The drawing under review shows one solid part. Ordinate dimensions are in mm from its lowest x, y, z. A direction names the side the tool comes from. Round coordinates to 2 decimals unless told otherwise and drop trailing zeros. Write each loop counter-clockwise with the first axis right and the second up, starting at its lowest first coordinate (ties: lowest second). Pieces come first, ordered by that corner, then holes.
Item 1: Machinability: for the marked faces 1 and 2, which of the approach directions +Z, -Z, +X, -X, +Y, -Y give a long, thin tool a straight path to every point of the face, cutting with its end or side? Answer none if there is none.
Item 2: Draft analysis for pull direction X (two halves, no side actions). For the marked faces 3, 4 and 5, state which applies: +X half, -X half, draft (parallel to the pull), parting line (faces both ways), or undercut.
Item 3: Clearance check with a flat-ended pin moving along its axis: pin 1 Ø0.8 at (y, z) = (12, 1.5) entering from +X. State where the tip first meets the part, or that it passes through.
Item 4: To check wall thickness, follow L1, parallel to Y at x = 4.5, z = 1.45; L2, parallel to Y at x = 4, z = 2; L3, parallel to X at y = 16.5, z = 1.35. State the ranges of each line that lie inside material, in increasing order.
Item 5: Add section A-A (x = 2.5). Give the boundary of the cut face in (y, z).
Item 6: Add section C-C (y = 14.5). Give the boundary of the cut face in (x, z).
Item 7: Add section B-B (z = 1.35). Give the boundary of the cut face in (x, y) (3 decimals).
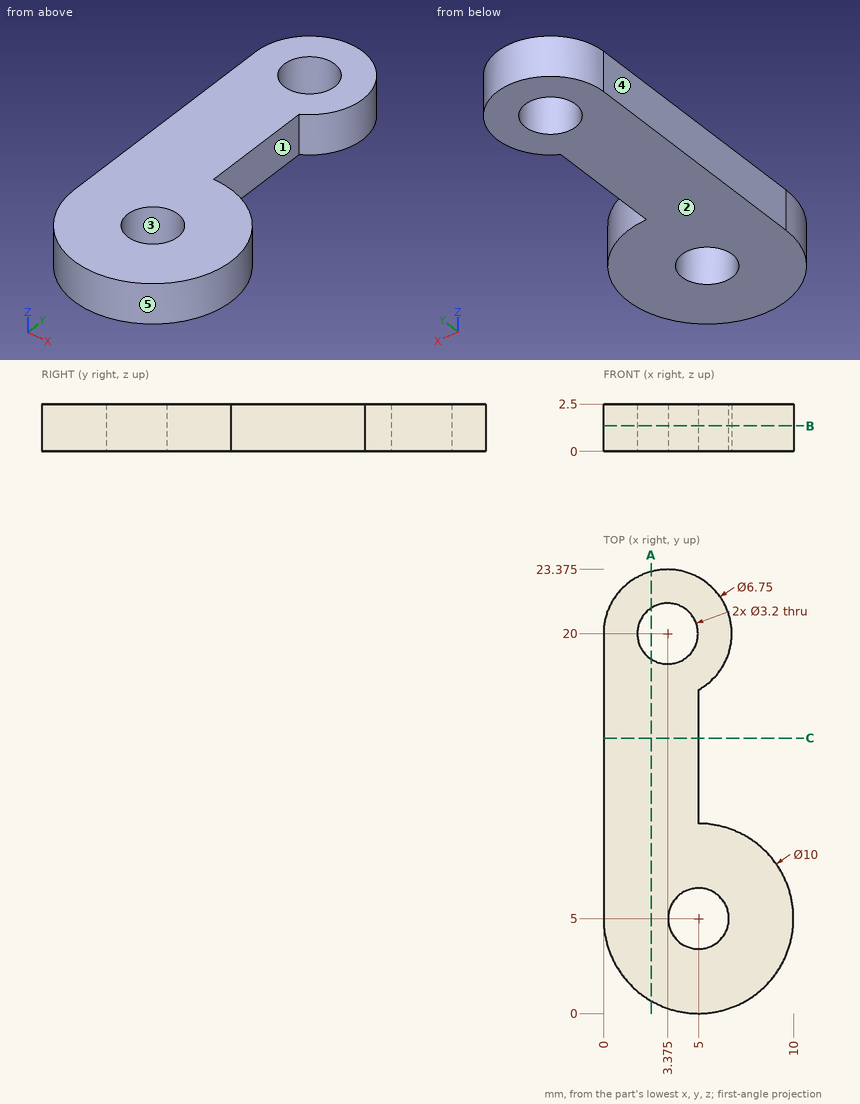
Numbers:
1. face 1: +Z, -Z, +X
1. face 2: -Z, +X, -X, +Y, -Y
2. face 3: undercut
2. face 4: -X half
2. face 5: parting line
3. pin 1: stops at x = 5
4. L1: y = 0.03 to 3.48, 6.52 to 18.86, 21.14 to 23.18
4. L2: y = 0.1 to 3.75, 6.25 to 18.53, 21.47 to 23.32
4. L3: x = 0 to 5
5. outline: (0.67, 0) - (18.66, 0) - (18.66, 2.5) - (0.67, 2.5) - close; (21.34, 0) - (23.26, 0) - (23.26, 2.5) - (21.34, 2.5) - close
6. outline: (0, 0) - (5, 0) - (5, 2.5) - (0, 2.5) - close
7. outline: (0, 5) arc R5 ccw (long way) to (5, 10) - (5, 17.042) arc R3.375 ccw (long way) to (0, 20) - close; hole circle Ø3.2 at (3.375, 20); hole circle Ø3.2 at (5, 5)
